from build123d import *

# Parameters (mm, degrees)
SKETCH1_R               = 4
BOSS_EXTRUDE1_DEPTH     = 5
CUT_EXTRUDE1_DEPTH      = 6.0000001
BOSS_EXTRUDE3_DEPTH     = 5
SKETCH7_R               = 1.5
CUT_EXTRUDE2_DEPTH      = 3.373709786
CUT_EXTRUDE2_DEPTH_BACK = 14.626290414


with BuildPart() as part:
    # Sketch1 → Boss-Extrude1 (new body)
    with BuildSketch(Plane(origin=(0, 0, 0), x_dir=(1, 0, 0), z_dir=(0, 1, 0))):
        with BuildLine():
            Line((-2.5, 8), (31.690345961, 5.462833873))
            add(Edge.make_bspline(
                [(31.690345961, 5.462833873), (93.309654039, 0), (31.690345961, -5.462833873)],
                knots=[0, 0, 0, 1, 1, 1], degree=2))
            Line((31.690345961, -5.462833873), (-2.5, -8))
            ThreePointArc((-2.5, -8), (-10.5, 0), (-2.5, 8))
        make_face()
        with Locations((-2.5, 0)):
            Circle(SKETCH1_R, mode=Mode.SUBTRACT)
    extrude(amount=BOSS_EXTRUDE1_DEPTH)

    # Sketch5 → Cut-Extrude1 (cut, through all)
    with BuildSketch(Plane(origin=(0, 5, 0), x_dir=(1, 0, 0), z_dir=(0, 1, 0))):
        with BuildLine():
            Line((1.372805365, -1.000689064), (3.672323333, -1.000689064))
            ThreePointArc((3.672323333, -1.000689064), (4.673012397, 0), (3.672323333, 1.000689064))
            Line((3.672323333, 1.000689064), (1.372805365, 1.000689064))
            ThreePointArc((1.372805365, 1.000689064), (1.5, 0), (1.372805365, -1.000689064))
        make_face()
        with BuildLine():
            Line((-6.372983346, 1), (-10.437253933, 1))
            ThreePointArc((-10.437253933, 1), (-10.5, 0), (-10.437253933, -1))
            Line((-10.437253933, -1), (-6.372983346, -1))
            ThreePointArc((-6.372983346, -1), (-6.5, 0), (-6.372983346, 1))
        make_face()
    extrude(amount=-CUT_EXTRUDE1_DEPTH, mode=Mode.SUBTRACT)

    # Sketch6 → Boss-Extrude3 (add)
    with BuildSketch(Plane(origin=(0, 5, 0), x_dir=(1, 0, 0), z_dir=(0, 1, 0))):
        with BuildLine():
            Line((-13.687253933, 1), (-10.437253933, 1))
            ThreePointArc((-10.437253933, 1), (-9.694264672, 3.498936386), (-8.187253933, 5.626290314))
            Line((-8.187253933, 5.626290314), (-13.687253933, 5.626290314))
            ThreePointArc((-13.687253933, 5.626290314), (-18.394261839, 0), (-13.687253933, -5.626290314))
            Line((-13.687253933, -5.626290314), (-8.187253933, -5.626290314))
            ThreePointArc((-8.187253933, -5.626290314), (-9.694264672, -3.498936386), (-10.437253933, -1))
            Line((-10.437253933, -1), (-13.687253933, -1))
            ThreePointArc((-13.687253933, -1), (-14.098831021, 0), (-13.687253933, 1))
        make_face()
    extrude(amount=-BOSS_EXTRUDE3_DEPTH)

    # Sketch7 → Cut-Extrude2 (cut, two sides)
    with BuildSketch(Plane(origin=(0, 0, -5.626290314), x_dir=(-1, 0, 0), z_dir=(0, 0, -1))) as cut_extrude2_sk:
        with Locations((10.937253933, 2.5)):
            Circle(SKETCH7_R)
    extrude(amount=CUT_EXTRUDE2_DEPTH, mode=Mode.SUBTRACT)
    extrude(cut_extrude2_sk.sketch, amount=-CUT_EXTRUDE2_DEPTH_BACK, mode=Mode.SUBTRACT)


solid = part.part
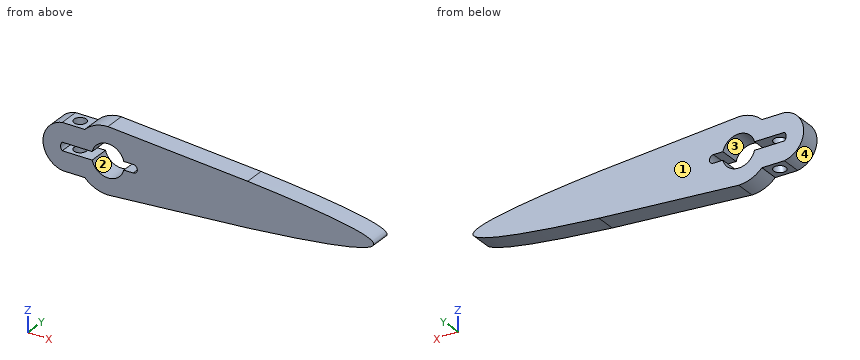
CAD build for the part. Positions are in the model's coordinates, mm. Face numbers are marked on the shaded views. Give positions to 0.01 mm unless a question says otherwise; leave off trailing zeros. Order: outer loops, then holes, each group sorted by start corner. A loop starts at its lowest first (then second) coordinate and runs counter-clockwise, first axis right, second up. Notation, with made-up numbers: (67, -35) - (84, -35) arc R30 ccw to (84, -10) - close; hole circle Ø7 at (55, 55.5). An arc over 180 degrees is marked (long way). Answer in a Markdown table with one row per item.
1. Probe probe 1 along X at (y, z) = (3.55, 0); probe 2 along Z at (x, y) = (29.5, 0.5); probe 3 along X at (y, z) = (4.3, 0.25). List the from-to ranges inside material, lowest first. Write a range as [from, to].
Data:
| item | result |
|---|---|
| probe 1 | x = [-18.39, -14.1], [4.67, 62.5] |
| probe 2 | z = [-5.63, 5.63] |
| probe 3 | x = [-18.39, -14.08], [4.64, 62.44] |
2. Saw through at A-A, the plane z = 3.25. Count the separate pieces of the cut face and the enclosed holes in it, plus the area to 3 significant figures.
Data:
| item | result |
|---|---|
| separate pieces | 2 |
| enclosed holes | 1 |
| area | 314 mm² |
3. Saw through at B-B, the plane x = 21. Give the cut face in (y, z).
Data:
| item | result |
|---|---|
| outline | (0, -6.26) - (5, -6.26) - (5, 6.26) - (0, 6.26) - close |
4. Flat gauge pins, fed straight in: pin 1 (1.8 mm diameter, centred on x = 2, y = 1.5, fed in from +Z); pin 2 (0.7 mm diameter, centred on x = 2.5, y = 2.5, fed in from -Z); pin 3 (2.5 mm diameter, centred on x = -10.94, y = 2.5, fed in from -Z). Where does each tip first touch, or does it go through?
Data:
| item | result |
|---|---|
| pin 1 | stops at z = 7.73 |
| pin 2 | stops at z = -7.65 |
| pin 3 | passes through |
5. Saw through at C-C, the plane x = 7.5. Give the cut face in (y, z).
Data:
| item | result |
|---|---|
| outline | (0, -7.26) - (5, -7.26) - (5, 7.26) - (0, 7.26) - close |
6. Pull direction Z, two halves, no side cores. Call the marked faces 1, 2, 3 and 4: pulls with the +Z half, pulls with the -Z half, needs draft (parallel to the pull), parting line crosses it, or undercut.
Data:
| item | result |
|---|---|
| face 1 | needs draft |
| face 2 | undercut |
| face 3 | undercut |
| face 4 | parting line crosses it |
